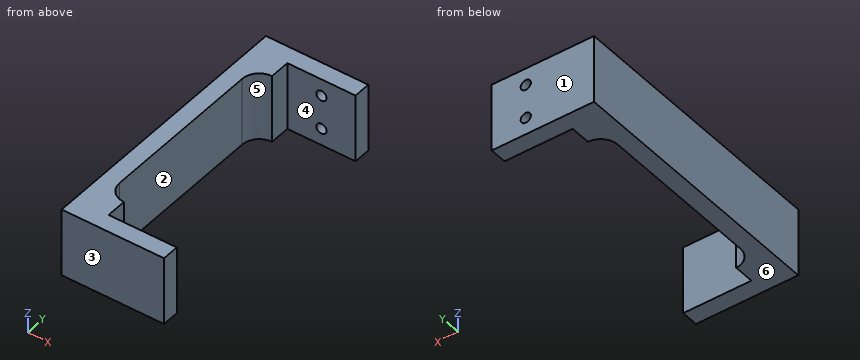
```python
from build123d import *

# Parameters (mm, degrees)
BOSS_EXTRUDE1_DEPTH = 20
BOSS_EXTRUDE2_DEPTH = 20
SKETCH4_R           = 1.5
CUT_EXTRUDE1_DEPTH  = 5


with BuildPart() as part:
    # Sketch1 → Boss-Extrude1 (new body)
    with BuildSketch(Plane.XY):
        Polygon((20, 0), (-10, 0), (-10, -80), (20, -80), (20, -75), (-5, -75), (-5, -5), (20, -5), align=None)
    extrude(amount=BOSS_EXTRUDE1_DEPTH)

    # Sketch3 → Boss-Extrude2 (add)
    with BuildSketch(Plane.XY):
        with BuildLine():
            Line((0, -5), (-5, -5))
            Line((-5, -5), (-5, -16))
            ThreePointArc((-5, -16), (-3.535533906, -12.464466094), (0, -11))
            Line((0, -11), (0, -5))
        make_face()
        with BuildLine():
            Line((-5, -75), (0, -75))
            Line((0, -75), (0, -69))
            ThreePointArc((0, -69), (-3.535533906, -67.535533906), (-5, -64))
            Line((-5, -64), (-5, -75))
        make_face()
    extrude(amount=BOSS_EXTRUDE2_DEPTH)

    # Sketch4 → Cut-Extrude1 (cut)
    with BuildSketch(Plane(origin=(0, 0, 0), x_dir=(1, 0, 0), z_dir=(0, 1, 0))):
        with Locations((10, -5)):
            Circle(SKETCH4_R)
        with Locations((10, -15)):
            Circle(SKETCH4_R)
    extrude(amount=-CUT_EXTRUDE1_DEPTH, mode=Mode.SUBTRACT)


solid = part.part
```
Design review of the part built by this model. Coordinates are the model's own, in mm. Face numbers are marked on the shaded views. A direction names the side the tool comes from. Round coordinates to 2 decimals unless told otherwise and drop trailing zeros. Order: outer loops, then holes, each group sorted by start corner. A loop starts at its lowest first (then second) coordinate and runs counter-clockwise, first axis right, second up. Notation, with made-up numbers: M 15.5,8 L 59.5,8 A14 ccw 59.5,34 Z; hole C 14,-7.75 d9. An arc over 180 degrees is marked long. Put each result on its own line as item: value.
Q1. Consider section D-D (z = 15). State the section outline as (x, y) points.
Reported:
outline: M -10,-80 L 20,-80 L 20,-75 L 0,-75 L 0,-69 A5 cw -5,-64 L -5,-16 A5 cw 0,-11 L 0,-5 L 8.5,-5 L 8.5,0 L -10,0 Z; M 11.5,-5 L 20,-5 L 20,0 L 11.5,0 Z
Q2. Insertion check: pin 1 Ø3.5 at (x, z) = (10, 15) entering from +Y. The pin has a flat end and moves straight along its axis. Give the tip position at first contact, or say it passes through.
Reported:
pin 1: y = 0
Q3. Consider section C-C (x = 6.5). State the section outline as (y, z) points.
Reported:
outline: M -80,0 L -75,0 L -75,20 L -80,20 Z; M -5,0 L 0,0 L 0,20 L -5,20 Z
Q4. Draft analysis for pull direction Y (two halves, no side actions). For the marked faces 3, 4, 5 and 6, state which applies: released by +Y, released by -Y, zero draft, split by the parting line, or undercut.
Reported:
face 3: released by -Y
face 4: undercut
face 5: undercut
face 6: zero draft
Q5. Consider section A-A (x = 10). State the section outline as (y, z) points, and give its area (3 significant figures).
Reported:
outline: M -80,0 L -75,0 L -75,20 L -80,20 Z; M -5,0 L 0,0 L 0,3.5 L -5,3.5 Z; M -5,6.5 L 0,6.5 L 0,13.5 L -5,13.5 Z; M -5,16.5 L 0,16.5 L 0,20 L -5,20 Z
area: 170 mm²
Q6. Consider section B-B (z = 2). State the section outline as (x, y) points.
Reported:
outline: M -10,-80 L 20,-80 L 20,-75 L 0,-75 L 0,-69 A5 cw -5,-64 L -5,-16 A5 cw 0,-11 L 0,-5 L 20,-5 L 20,0 L -10,0 Z
Q7. To check wall thickness, follow line 1 (Z direction, x = 10, y = -1.25); line 2 (Y direction, x = 10.25, z = 1.75); line 3 (X direction, y = -3.1, z = 15). State the ranges of each line that lie inside material, in increasing order.
Reported:
line 1: 0 to 3.5, 6.5 to 13.5, 16.5 to 20
line 2: -80 to -75, -5 to 0
line 3: -10 to 8.5, 11.5 to 20
Q8. Machinability: for the marked faces 1 and 2, which of the approach directions +Z, -Z, +X, -X, +Y, -Y give a long, thin tool a straight path to every point of the face, cutting with its end or side? Answer none if there is none.
Reported:
face 1: +Z, -Z, +X, -X, +Y
face 2: +Z, -Z, +X
